For this review, take the finished solid that the model builds, in its own axes (mm). Face numbers are marked on the shaded views. A direction names the side the tool comes from. Coordinates: 2 decimals unless noted, no trailing zeros. Loops run counter-clockwise (first coordinate to the right, second up) from the corner with the lowest first, then second, coordinate; pieces in that order, holes last. Notation, with made-up numbers: M -37.5,-26 L -26.5,-26 A19 ccw -26.5,6 Z; hole C 1,23 d9. An arc over 180 degrees is marked long. Put each result on its own line as item: value.
```python
from build123d import *

# Parameters (mm, degrees)
SKETCH_1_R          = 3.5
EXTRUDE_1_DEPTH     = 14
CUT_EXTRUDE_1_DEPTH = 7
SKETCH_3_W          = 1.9
SKETCH_3_H          = 1.5
SKETCH_3_W_2        = 1.5
SKETCH_3_H_2        = 1.9
CUT_EXTRUDE_2_DEPTH = 6
FILLET_2_R          = 0.1


with BuildPart() as part:
    # 草图1 → 凸台-拉伸1 (new body)
    with BuildSketch(Plane.XY):
        Circle(SKETCH_1_R)
    extrude(amount=EXTRUDE_1_DEPTH)

    # 草图2 → 切除-拉伸1 (cut)
    with BuildSketch(Plane.XY.offset(14)):
        with BuildLine():
            Line((1.469693846, 1.5), (-1.469693846, 1.5))
            ThreePointArc((-1.469693846, 1.5), (-0.8135241, -1.936021317), (2.1, 0))
            ThreePointArc((2.1, 0), (1.936021317, 0.8135241), (1.469693846, 1.5))
        make_face()
    extrude(amount=-CUT_EXTRUDE_1_DEPTH, mode=Mode.SUBTRACT)

    # 草图3 → 切除-拉伸2 (cut)
    with BuildSketch(Plane(origin=(0, 0, 0), x_dir=(-1, 0, 0), z_dir=(0, 0, -1))):
        with Locations((0, -1.7)):
            Rectangle(SKETCH_3_W, SKETCH_3_H)
        with Locations((1.7, 0)):
            Rectangle(SKETCH_3_W_2, SKETCH_3_H_2)
        Rectangle(SKETCH_3_W, SKETCH_3_H_2)
        with Locations((-1.7, 0)):
            Rectangle(SKETCH_3_W_2, SKETCH_3_H_2)
        with Locations((0, 1.7)):
            Rectangle(SKETCH_3_W, SKETCH_3_H)
    extrude(amount=-CUT_EXTRUDE_2_DEPTH, mode=Mode.SUBTRACT)

    # 圆角2
    fillet_2_edges = [part.edges().sort_by_distance(p)[0] for p in [
        (-0.95, -1.7, 6),
        (-0.95, -0.95, 3),
        (0, -2.45, 0),
        (-0.95, -2.45, 3),
        (0.95, -1.7, 0),
        (0.95, -2.45, 3),
        (1.7, -0.95, 6),
        (0.95, -0.95, 3),
        (2.45, 0, 0),
        (2.45, -0.95, 3),
        (1.7, 0.95, 0),
        (2.45, 0.95, 3),
        (0.95, 1.7, 0),
        (0.95, 0.95, 3),
        (0, 2.45, 6),
        (0.95, 2.45, 3),
        (-0.95, 1.7, 6),
        (-0.95, 2.45, 3),
        (-1.7, 0.95, 0),
        (-0.95, 0.95, 3),
        (-2.45, 0, 6),
        (-2.45, 0.95, 3),
        (-1.7, -0.95, 6),
        (-2.45, -0.95, 3),
        (0, -2.45, 6),
        (0.95, -1.7, 6),
        (2.45, 0, 6),
        (1.7, 0.95, 6),
        (0.95, 1.7, 6),
        (-1.7, 0.95, 6),
        (-0.95, -1.7, 0),
        (-1.7, -0.95, 0),
        (-2.45, 0, 0),
        (-0.95, 1.7, 0),
        (0, 2.45, 0),
        (1.7, -0.95, 0),
    ]]
    fillet(fillet_2_edges, radius=FILLET_2_R)


solid = part.part
```
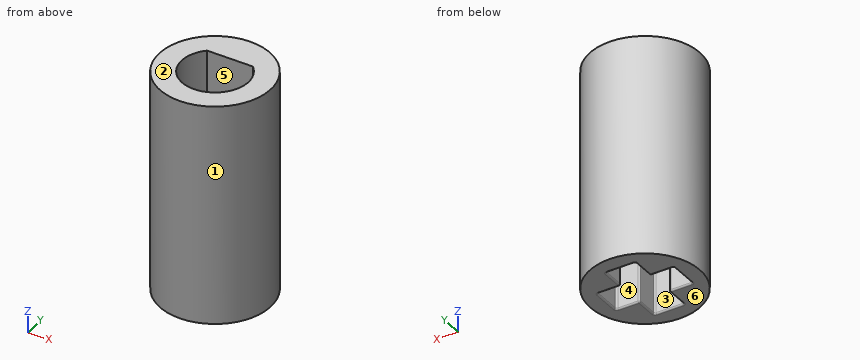
(1) Tool access review of the marked faces 4, 5 and 6: name each direction out of +Z, -Z, +X, -X, +Y, -Y from which nothing blocks a thin tool from reaching the whole face with its end or side.
Determined:
face 4: -Z
face 5: +Z
face 6: -Z, +X, -X, +Y, -Y
(2) Add section D-D (z = 10.75). Write out the cut boundary in (x, y), plus the area to 3 significant figures.
Determined:
outline: C 0,0 d7; hole M -1.47,1.5 A2.1 ccw long 1.47,1.5 Z
area: 25.8 mm^2
(3) Wall thickness on line 1 along Y through (x, z) = (0, 12.25); line 2 along Z through (x, y) = (1.25, 1.25); line 3 along X through (y, z) = (-1.5, 9): over which ranges is each line inside the solid? List them lowest first. Write a range as [from, to].
Determined:
line 1: y = [-3.5, -2.1], [1.5, 3.5]
line 2: z = [0, 7]
line 3: x = [-3.16, -1.47], [1.47, 3.16]
(4) For pin 1 (1.8 mm diameter, centred on x = 0, y = -1, fed in from +Z); pin 2 (1.5 mm diameter, centred on y = -1, z = 12, fed in from -X); pin 3 (0.5 mm diameter, centred on x = -0.5, z = 4.5, fed in from -Y), all flat-tipped, find the tip position at first contact; note any pin that passes through.
Determined:
pin 1: stops at z = 7
pin 2: stops at x = -3.49
pin 3: stops at y = -3.49
(5) Draft analysis for pull direction Y (two halves, no side actions). For the marked faces 1, 2 and 3, state which applies: +Y half, -Y half, draft (parallel to the pull), parting line (faces both ways), or undercut.
Determined:
face 1: parting line
face 2: draft
face 3: undercut
(6) Add section C-C (y = 0.25). Write out the cut boundary in (x, z).
Determined:
outline: M -3.49,0 L -2.55,0 A0.1 ccw -2.45,0.1 L -2.45,5.9 A0.1 cw -2.35,6 L 2.35,6 A0.1 cw 2.45,5.9 L 2.45,0.1 A0.1 ccw 2.55,0 L 3.49,0 L 3.49,14 L 2.09,14 L 2.09,7 L -2.09,7 L -2.09,14 L -3.49,14 Z
(7) Add section A-A (z = 5). Write out the cut boundary in (x, y), plus the area to 3 significant figures.
Determined:
outline: C 0,0 d7; hole M -2.45,-0.85 A0.1 ccw -2.35,-0.95 L -1.05,-0.95 A0.1 cw -0.95,-1.05 L -0.95,-2.35 A0.1 ccw -0.85,-2.45 L 0.85,-2.45 A0.1 ccw 0.95,-2.35 L 0.95,-1.05 A0.1 cw 1.05,-0.95 L 2.35,-0.95 A0.1 ccw 2.45,-0.85 L 2.45,0.85 A0.1 ccw 2.35,0.95 L 1.05,0.95 A0.1 cw 0.95,1.05 L 0.95,2.35 A0.1 ccw 0.85,2.45 L -0.85,2.45 A0.1 ccw -0.95,2.35 L -0.95,1.05 A0.1 cw -1.05,0.95 L -2.35,0.95 A0.1 ccw -2.45,0.85 Z
area: 23.5 mm^2
(8) Add section B-B (x = 0). Write out the cut boundary in (y, z), plus the area to 3 significant figures.
Determined:
outline: M -3.5,0 L -2.55,0 A0.1 ccw -2.45,0.1 L -2.45,5.9 A0.1 cw -2.35,6 L 2.35,6 A0.1 cw 2.45,5.9 L 2.45,0.1 A0.1 ccw 2.55,0 L 3.5,0 L 3.5,14 L 1.5,14 L 1.5,7 L -2.1,7 L -2.1,14 L -3.5,14 Z
area: 43.4 mm^2
